Design review of the part built by this model. Coordinates are the model's own, in mm. A direction names the side the tool comes from. Round coordinates to 2 decimals unless told otherwise and drop trailing zeros. Order: outer loops, then holes, each group sorted by start corner. A loop starts at its lowest first (then second) coordinate and runs counter-clockwise, first axis right, second up. Notation, with made-up numbers: M 32.5,-16 L 89.5,-16 A13 cw 89.5,8 Z; hole C -0.75,4.5 d8. An arc over 180 degrees is marked long. Use a Markdown table: item, result. Add a question column.
(1) Take a section at B-B (y = 51). Write out the cut boundary in (x, z), then the cut area to 3 significant figures.
(2) Machinability: for faces 1 (the face through (-12.7, -5, 2)), 2 (the face through (-34, 26.131, 30)), 3 (the face through (-34, 13.431, 38)), 4 (the face through (-35, -35.23, 30)), which of the approach directions +Z, -Z, +X, -X, +Y, -Y give a long, thin tool a straight path to every point of the face, cutting with its end or side? Answer none if there is none.
(3) To check wall thickness, follow probe 1 along Y at (x, z) = (-33.5, -8); probe 2 along Y at (x, z) = (-29, 28.5); probe 3 along Z at (x, y) = (-8.5, 32). State the ranges of each line that lie inside material, in increasing order. Write a range as from..to.
(4) Take a section at D-D (z = 9). Write out the cut boundary in (x, y).
(5) The part is to be moulded in two halves that separate along Y. For faces 5 (the face through (-35, -22.53, 38)), 6 (the face through (-33.59, 80.59, -12.52)), 7 (the face through (-55.994, -4, 2)), say which applies: released by +Y, released by -Y, zero draft, split by the parting line, or undercut.
(6) For pin 1 (6 mm diameter, centred on x = -25, z = 8, fed in from +Y); pin 2 (20.5 mm diameter, centred on x = -51.5, y = 16, fed in from +Z); pin 3 (13 mm diameter, centred on x = -28.5, z = 32.5, fed in from -Y); pin 4 (9 mm diameter, centred on x = -34.35, z = 43.51, fed in from +Y), all flat-tipped, find the tip position at first contact; note any pin that passes through.
(7) Take a section at C-C (x = -26.5). Write out the cut boundary in (y, z), then the cut area to 3 significant figures.
```python
from build123d import *

# Parameters (mm, degrees)
F0_R     = 12.7
F1_DEPTH = 25.4
F3_DEPTH = 38.1
F5_DEPTH = 69.088
F7_R     = 5.08
F8_DEPTH = 12.7
F6_R     = 5.08
F9_DEPTH = 12.7


# Not quite as in the source:
# - a feature names something its author has since deleted; it is built from what else it names


with BuildPart() as f1:
    # F0 (on Top) → F1 (new body)
    with BuildSketch(Plane.XY):
        with BuildLine():
            Line((0, -55.3492553601), (0, 0))
            Line((0, 0), (0, 46.2507446399))
            ThreePointArc((0, 46.2507446399), (-34.3468652373, 80.5976098772), (-68.6937304746, 46.2507446399))
            Line((-68.6937304746, 46.2507446399), (-68.6937304746, -55.3492553601))
            ThreePointArc((-68.6937304746, -55.3492553601), (-34.3468652373, -89.6961205974), (0, -55.3492553601))
        make_face()
        with Locations((-34.3468652373, -55.3492553601)):
            Circle(F0_R, mode=Mode.SUBTRACT)
        with Locations((-34.3468652373, 46.2507446399)):
            Circle(F0_R, mode=Mode.SUBTRACT)
    extrude(amount=-F1_DEPTH)

    # F2 (on face) → F3 (join)
    with BuildSketch(Plane.XY):
        Polygon((-55.9937304746, 26.1313845437), (-55.9937304746, -4.5492553601), (-55.9937304746, -35.2298952639), (-12.7, -35.2298952639), (-12.7, -4.5492553601), (-12.7, 26.1313845437), align=None)
    extrude(amount=F3_DEPTH)

    # F4 (on face) → F5 (cut)
    with BuildSketch(Plane.YZ.offset(-12.7)):
        with BuildLine():
            Line((13.4313845437, 38.1), (-22.5298952639, 38.1))
            Line((-22.5298952639, 38.1), (-22.5298952639, 15.044502914))
            ThreePointArc((-22.5298952639, 15.044502914), (-4.5492553601, 2.5536219989), (13.4313845437, 15.044502914))
            Line((13.4313845437, 15.044502914), (13.4313845437, 38.1))
        make_face()
    extrude(amount=-F5_DEPTH, mode=Mode.SUBTRACT)

    # F7 (on face) → F8 (join)
    with BuildSketch(Plane(origin=(0, 26.1313845437, 0), x_dir=(-1, 0, 0), z_dir=(0, 1, 0))):
        with BuildLine():
            Line((12.7, 38.1), (55.9937304746, 38.1))
            ThreePointArc((55.9937304746, 38.1), (34.3468652373, 59.7468652373), (12.7, 38.1))
        make_face()
        with Locations((34.3468652373, 43.5117163093)):
            Circle(F7_R, mode=Mode.SUBTRACT)
    extrude(amount=-F8_DEPTH)

    # F6 (on face) → F9 (join)
    with BuildSketch(Plane.XZ.offset(35.2298952639)):
        with BuildLine():
            Line((-55.9937304746, 38.1), (-12.7, 38.1))
            ThreePointArc((-12.7, 38.1), (-34.3468652373, 59.7468652373), (-55.9937304746, 38.1))
        make_face()
        with Locations((-34.3468652373, 43.5117163093)):
            Circle(F6_R, mode=Mode.SUBTRACT)
    extrude(amount=-F9_DEPTH)


solid = f1.part
```
Verdict:
| question | item | result |
|---|---|---|
| 1 | outline | M -68.36,-25.4 L -46.13,-25.4 L -46.13,0 L -68.36,0 Z; M -22.57,-25.4 L -0.33,-25.4 L -0.33,0 L -22.57,0 Z |
| 1 | area | 1,130 mm^2 |
| 2 | face 1 | +Z, +X, +Y, -Y |
| 2 | face 2 | +Z, +X, -X, +Y |
| 2 | face 3 | +Z, +X, -X |
| 2 | face 4 | +Z, +X, -X, -Y |
| 3 | probe 1 | y = -89.69..-68.02, -42.68..33.58, 58.92..80.59 |
| 3 | probe 2 | y = -35.23..-22.53, 13.43..26.13 |
| 3 | probe 3 | z = -25.4..0 |
| 4 | outline | M -55.99,-35.23 L -12.7,-35.23 L -12.7,-18.9 L -55.99,-18.9 Z; M -55.99,9.8 L -12.7,9.8 L -12.7,26.13 L -55.99,26.13 Z |
| 5 | face 5 | undercut |
| 5 | face 6 | released by +Y |
| 5 | face 7 | zero draft |
| 6 | pin 1 | stops at y = 26.13 |
| 6 | pin 2 | stops at z = 58.62 |
| 6 | pin 3 | stops at y = -35.23 |
| 6 | pin 4 | passes through |
| 7 | outline | M -88.79,-25.4 L -65.34,-25.4 L -65.34,0 L -88.79,0 Z; M -45.36,-25.4 L 36.26,-25.4 L 36.26,0 L 26.13,0 L 26.13,58.27 L 13.43,58.27 L 13.43,15.04 A19.19 cw -22.53,15.04 L -22.53,58.27 L -35.23,58.27 L -35.23,0 L -45.36,0 Z; M 56.24,-25.4 L 79.69,-25.4 L 79.69,0 L 56.24,0 Z |
| 7 | area | 4,960 mm^2 |
